Autodesk Inventor part; units mm, degrees
ref_plane "YZ Plane" through (0, 0, 0) normal (1, 0, 0) x (0, 1, 0)
ref_plane "XZ Plane" through (0, 0, 0) normal (0, 1, 0) x (-1, 0, 0)
ref_plane "XY Plane" through (0, 0, 0) normal (0, 0, 1) x (1, 0, 0)
sketch "Sketch1" plane through (0, 0, 0) normal (0, 0, 1) x (1, 0, 0)
  arc A0 (0, -0.381) -> (11, 10.619) centre (0, 10.619) ccw
  line L0 (11, 99.379) -> (11, 10.619)
  line L1 (0, -0.381) -> (-170.96, -0.381)
  arc A1 (11, 99.379) -> (0, 110.379) centre (0, 99.379) ccw
  line L2 (-170.96, 110.379) -> (0, 110.379)
  arc A2 (-170.96, 110.379) -> (-181.96, 99.379) centre (-170.96, 99.379) ccw
  line L3 (-181.96, 10.619) -> (-181.96, 99.379)
  arc A3 (-181.96, 10.619) -> (-170.96, -0.381) centre (-170.96, 10.619) ccw
  circle A4 centre (-22.38, 21.199) radius 1.5
  circle A5 centre (-148.58, 21.199) radius 1.5
  circle A6 centre (-148.58, 86.849) radius 1.5
  circle A7 centre (-22.38, 86.849) radius 1.5
  circle A8 centre (-22.38, 21.199) radius 1.905
  circle A9 centre (-22.38, 86.849) radius 1.905
  line L4 (-41.31, 1.719) -> (-129.65, 1.719)
  line L5 (-129.65, 108.279) -> (-41.31, 108.279)
  line L6 (8.9, 71.419) -> (8.9, 36.009)
  line L7 (-34.96, 23.309) -> (-34.96, 8.069)
  line L8 (-28.61, 29.659) -> (2.55, 29.659)
  arc A10 (-28.61, 29.659) -> (-34.96, 23.309) centre (-28.61, 23.309) ccw
  line L9 (2.55, 77.769) -> (-28.61, 77.769)
  line L10 (-34.96, 84.119) -> (-34.96, 101.929)
  arc A11 (-34.96, 84.119) -> (-28.61, 77.769) centre (-28.61, 84.119) ccw
  arc A12 (2.55, 29.659) -> (8.9, 36.009) centre (2.55, 36.009) ccw
  arc A13 (-41.31, 1.719) -> (-34.96, 8.069) centre (-41.31, 8.069) ccw
  arc A14 (-34.96, 101.929) -> (-41.31, 108.279) centre (-41.31, 101.929) ccw
  arc A15 (8.9, 71.419) -> (2.55, 77.769) centre (2.55, 71.419) ccw
  line L11 (-29.88, 25.199) -> (-29.88, 17.199)
  line L12 (-14.88, 25.199) -> (-29.88, 25.199)
  line L13 (-29.88, 82.849) -> (-14.88, 82.849)
  line L14 (-29.88, 90.849) -> (-29.88, 82.849)
  circle A16 centre (-148.58, 21.199) radius 1.905
  circle A17 centre (-148.58, 86.849) radius 1.905
  line L15 (-179.86, 71.419) -> (-179.86, 36.009)
  line L16 (-136, 23.309) -> (-136, 8.069)
  line L17 (-142.35, 29.659) -> (-173.51, 29.659)
  arc A18 (-136, 23.309) -> (-142.35, 29.659) centre (-142.35, 23.309) ccw
  line L18 (-173.51, 77.769) -> (-142.35, 77.769)
  line L19 (-136, 84.119) -> (-136, 101.929)
  arc A19 (-142.35, 77.769) -> (-136, 84.119) centre (-142.35, 84.119) ccw
  arc A20 (-179.86, 36.009) -> (-173.51, 29.659) centre (-173.51, 36.009) ccw
  arc A21 (-136, 8.069) -> (-129.65, 1.719) centre (-129.65, 8.069) ccw
  arc A22 (-129.65, 108.279) -> (-136, 101.929) centre (-129.65, 101.929) ccw
  arc A23 (-173.51, 77.769) -> (-179.86, 71.419) centre (-173.51, 71.419) ccw
  point P0 (0, 0)
  point P1 (-34.96, 1.719)
  point P2 (8.9, 29.659)
  point P3 (8.9, 77.769)
  point P4 (-34.96, 77.769)
  point P5 (-34.96, 108.279)
  dimension "d1" = 23.53
  dimension "d2" = 3.81
  dimension "d5" = 3.81
  dimension "d16" = 27.94
  dimension "d18" = 6.35
  dimension "d21" = 6.35
  dimension "d22" = 6.35
  dimension "d23" = 2.1
  dimension "d24" = 2.1
  dimension "d25" = 2.1
  dimension "d33" = 5.08
  dimension "d34" = 5.08
  dimension "d35" = 5.08
  dimension "d36" = 6.35
  dimension "d37" = 6.35
extrude "Extrusion3" add sketch "Sketch1" along normal blind 2.1 contours L1 A3 L3 A2 L2 A1 L0 A0
sketch "Sketch4" plane through (0, 0, 2.1) normal (0, 0, 1) x (1, 0, 0)
  arc A0 (-28.61, 29.659) -> (-34.96, 23.309) centre (-28.61, 23.309) ccw
  line L0 (-34.96, 23.309) -> (-34.96, 8.069)
  arc A1 (-41.31, 1.719) -> (-34.96, 8.069) centre (-41.31, 8.069) ccw
  line L1 (-41.31, 1.719) -> (-129.65, 1.719)
  arc A2 (-136, 8.069) -> (-129.65, 1.719) centre (-129.65, 8.069) ccw
  line L2 (-136, 8.069) -> (-136, 23.309)
  arc A3 (-136, 23.309) -> (-142.35, 29.659) centre (-142.35, 23.309) ccw
  line L3 (-142.35, 29.659) -> (-173.51, 29.659)
  arc A4 (-179.86, 36.009) -> (-173.51, 29.659) centre (-173.51, 36.009) ccw
  line L4 (-179.86, 36.009) -> (-179.86, 71.419)
  arc A5 (-173.51, 77.769) -> (-179.86, 71.419) centre (-173.51, 71.419) ccw
  line L5 (-173.51, 77.769) -> (-142.35, 77.769)
  arc A6 (-142.35, 77.769) -> (-136, 84.119) centre (-142.35, 84.119) ccw
  line L6 (-136, 84.119) -> (-136, 101.929)
  arc A7 (-129.65, 108.279) -> (-136, 101.929) centre (-129.65, 101.929) ccw
  line L7 (-129.65, 108.279) -> (-41.31, 108.279)
  arc A8 (-34.96, 101.929) -> (-41.31, 108.279) centre (-41.31, 101.929) ccw
  line L8 (-34.96, 101.929) -> (-34.96, 84.119)
  arc A9 (-34.96, 84.119) -> (-28.61, 77.769) centre (-28.61, 84.119) ccw
  line L9 (-28.61, 77.769) -> (2.55, 77.769)
  arc A10 (8.9, 71.419) -> (2.55, 77.769) centre (2.55, 71.419) ccw
  line L10 (8.9, 71.419) -> (8.9, 36.009)
  arc A11 (2.55, 29.659) -> (8.9, 36.009) centre (2.55, 36.009) ccw
  line L11 (2.55, 29.659) -> (-28.61, 29.659)
  circle A12 centre (-148.58, 86.849) radius 1.905
  circle A13 centre (-148.58, 21.199) radius 1.905
  circle A14 centre (-22.38, 86.849) radius 1.905
  circle A15 centre (-22.38, 21.199) radius 1.905
  arc A16 (0, -0.381) -> (11, 10.619) centre (0, 10.619) ccw
  line L12 (11, 10.619) -> (11, 99.379)
  arc A17 (11, 99.379) -> (0, 110.379) centre (0, 99.379) ccw
  line L13 (0, 110.379) -> (-170.96, 110.379)
  arc A18 (-170.96, 110.379) -> (-181.96, 99.379) centre (-170.96, 99.379) ccw
  line L14 (-181.96, 99.379) -> (-181.96, 10.619)
  arc A19 (-181.96, 10.619) -> (-170.96, -0.381) centre (-170.96, 10.619) ccw
  line L15 (-170.96, -0.381) -> (0, -0.381)
  arc A20 (0, 1.719) -> (8.9, 10.619) centre (0, 10.619) ccw
  line L16 (8.9, 10.619) -> (8.9, 99.379)
  arc A21 (8.9, 99.379) -> (0, 108.279) centre (0, 99.379) ccw
  line L17 (0, 108.279) -> (-170.96, 108.279)
  arc A22 (-170.96, 108.279) -> (-179.86, 99.379) centre (-170.96, 99.379) ccw
  line L18 (-179.86, 99.379) -> (-179.86, 10.619)
  arc A23 (-179.86, 10.619) -> (-170.96, 1.719) centre (-170.96, 10.619) ccw
  line L19 (-170.96, 1.719) -> (0, 1.719)
  point P0 (0, 0)
  dimension "d40" = 2.1
extrude "Extrusion4" add sketch "Sketch4" along normal blind 8.5 contours L15 A19 L14 A18 L13 A17 L12 A16
ref_plane "Work Plane1" through (-85.48, 10.619, 10.6) normal (-1, 0, 0) x (0, 0, 1)
ref_plane "Work Plane2" through (-170.96, 54.999, 10.6) normal (0, -1, 0) x (1, 0, 0)
sketch "Sketch9" plane through (0, 0, 0) normal (0, 0, -1) x (-1, 0, 0)
  arc A0 (-8.9, 10.619) -> (0, 1.719) centre (0, 10.619) ccw
  arc A1 (-6.8, 10.619) -> (0, 3.819) centre (0, 10.619) ccw
  line L0 (0, 1.719) -> (0, 3.819)
  line L1 (-6.8, 10.619) -> (-8.9, 10.619)
  arc A2 (170.96, 1.719) -> (179.86, 10.619) centre (170.96, 10.619) ccw
  arc A3 (170.96, 3.819) -> (177.76, 10.619) centre (170.96, 10.619) ccw
  line L2 (170.96, 3.819) -> (170.96, 1.719)
  line L3 (179.86, 10.619) -> (177.76, 10.619)
  arc A4 (179.86, 99.379) -> (170.96, 108.279) centre (170.96, 99.379) ccw
  arc A5 (177.76, 99.379) -> (170.96, 106.179) centre (170.96, 99.379) ccw
  line L4 (177.76, 99.379) -> (179.86, 99.379)
  line L5 (170.96, 108.279) -> (170.96, 106.179)
  arc A6 (0, 106.179) -> (-6.8, 99.379) centre (0, 99.379) ccw
  arc A7 (0, 108.279) -> (-8.9, 99.379) centre (0, 99.379) ccw
  line L6 (-8.9, 99.379) -> (-6.8, 99.379)
  line L7 (0, 106.179) -> (0, 108.279)
  line L8 (170.96, 1.719) -> (0, 1.719)
  line L9 (0.508, 1.719) -> (0, 1.719)
  line L10 (-6.36, 11.127) -> (-8.9, 11.127)
  line L11 (-8.9, 11.127) -> (-8.9, 10.619)
  line L12 (0.508, 1.719) -> (0.508, 4.259)
  arc A8 (-6.36, 11.127) -> (0.508, 4.259) centre (0.748, 11.367) ccw
  arc A9 (-8.9, 10.619) -> (0, 1.719) centre (0, 10.619) ccw
  line L13 (-6.36, 98.871) -> (-8.9, 98.871)
  line L14 (-8.9, 99.379) -> (-8.9, 10.619)
  line L15 (0.508, 105.739) -> (0.508, 108.279)
  line L16 (0.508, 108.279) -> (0, 108.279)
  arc A10 (0, 108.279) -> (-8.9, 98.871) centre (0, 99.3653) ccw
  arc A11 (0.508, 105.739) -> (-6.36, 98.871) centre (0.748, 98.631) ccw
  line L17 (0, -0.381) -> (170.96, -0.381)
  line L18 (85.48, -0.381) -> (85.48, 110.379)
  line L19 (170.96, 110.379) -> (0, 110.379)
  arc A12 (170.96, 1.719) -> (179.86, 10.619) centre (170.96, 10.619) ccw
  line L20 (170.452, 1.719) -> (170.96, 1.719)
  line L21 (177.32, 11.127) -> (179.86, 11.127)
  line L22 (170.452, 1.719) -> (170.452, 4.259)
  arc A13 (170.452, 4.259) -> (177.32, 11.127) centre (170.212, 11.367) ccw
  line L23 (177.32, 98.871) -> (179.86, 98.871)
  line L24 (179.86, 99.379) -> (179.86, 10.619)
  line L25 (170.452, 105.739) -> (170.452, 108.279)
  line L26 (170.452, 108.279) -> (170.96, 108.279)
  arc A14 (179.86, 98.871) -> (170.96, 108.279) centre (170.96, 99.3653) ccw
  arc A15 (177.32, 98.871) -> (170.452, 105.739) centre (170.212, 98.631) ccw
  point P0 (0, 0)
  point P1 (17.526, 1.719)
  dimension "d73" = 0.508
  dimension "d74" = 0.508
  dimension "d75" = 2.54
  dimension "d76" = 2.54
  dimension "d77" = 7.112
  dimension "d78" = 2.54
  dimension "d79" = 2.54
  dimension "d80" = 0.508
  dimension "d81" = 0.508
  dimension "d82" = 7.112
extrude "Extrusion7" cut sketch "Sketch9" against normal up to next contours L1 A1 L0 A0 | L7 A6 L6 A7 | A10 L16 L15 A11 L13 | L23 A15 L25 L26 L5 A5 L4 L24 | L24 A4 A14 | L22 A13 L21 L24 L3 A3 L2 L8 | L2 A3 L3 A2 | L4 A5 L5 A4
sketch "Sketch10" plane through (0, 0, 0) normal (0, 0, -1) x (-1, 0, 0)
  line L0 (-3.38, 18.0763) -> (14.4, 27.559)
  line L1 (14.4, 27.559) -> (-3.38, 27.559)
  line L2 (-3.38, 27.559) -> (-3.38, 18.0763)
  line L3 (10.7529, 7.239) -> (29.8029, 17.399)
  line L4 (29.8029, 17.399) -> (29.8029, 7.239)
  line L5 (29.8029, 7.239) -> (10.7529, 7.239)
  line L6 (0, -0.381) -> (170.96, -0.381)
  line L7 (-11, 99.379) -> (-11, 10.619)
  line L8 (181.96, 99.379) -> (181.96, 10.619)
  line L9 (181.96, 54.999) -> (-11, 54.999)
  line L10 (-11, 10.619) -> (-11, 99.379)
  line L11 (85.48, -0.381) -> (85.48, 110.379)
  line L12 (0, 110.379) -> (170.96, 110.379)
  line L13 (174.34, 18.0763) -> (156.56, 27.559)
  line L14 (156.56, 27.559) -> (174.34, 27.559)
  line L15 (174.34, 27.559) -> (174.34, 18.0763)
  line L16 (160.2071, 7.239) -> (141.1571, 17.399)
  line L17 (141.1571, 17.399) -> (141.1571, 7.239)
  line L18 (141.1571, 7.239) -> (160.2071, 7.239)
  line L19 (-3.38, 91.9217) -> (14.4, 82.439)
  line L20 (14.4, 82.439) -> (-3.38, 82.439)
  line L21 (-3.38, 82.439) -> (-3.38, 91.9217)
  line L22 (10.7529, 102.759) -> (29.8029, 92.599)
  line L23 (29.8029, 92.599) -> (29.8029, 102.759)
  line L24 (29.8029, 102.759) -> (10.7529, 102.759)
  line L25 (141.1571, 102.759) -> (160.2071, 102.759)
  line L26 (141.1571, 92.599) -> (141.1571, 102.759)
  line L27 (160.2071, 102.759) -> (141.1571, 92.599)
  line L28 (174.34, 91.9217) -> (156.56, 82.439)
  line L29 (156.56, 82.439) -> (174.34, 82.439)
  line L30 (174.34, 82.439) -> (174.34, 91.9217)
  point P0 (0, 0)
  point P1 (-11, 19.255)
  dimension "d85" = 17.78
  dimension "d86" = 19.05
  dimension "d87" = 10.16
  dimension "d88" = 7.62
  dimension "d89" = 7.62
  dimension "d102" = 27.94
extrude "Extrusion8" cut sketch "Sketch10" against normal up to next
sketch "Sketch11" plane through (0, 0, 2.1) normal (0, 0, 1) x (1, 0, 0)
  arc A0 (-144.389, 84.944) -> (-144.389, 88.754) centre (-144.389, 86.849) ccw
  circle A1 centre (-148.58, 86.849) radius 1.905
  arc A2 (-152.771, 88.754) -> (-152.771, 84.944) centre (-152.771, 86.849) ccw
  line L0 (-152.771, 88.754) -> (-144.389, 88.754)
  line L1 (-144.389, 84.944) -> (-152.771, 84.944)
  circle A3 centre (-148.58, 21.199) radius 1.905
  arc A4 (-144.389, 19.294) -> (-144.389, 23.104) centre (-144.389, 21.199) ccw
  arc A5 (-152.771, 23.104) -> (-152.771, 19.294) centre (-152.771, 21.199) ccw
  line L2 (-152.771, 23.104) -> (-144.389, 23.104)
  line L3 (-152.771, 19.294) -> (-144.389, 19.294)
  line L4 (-85.48, -22.533) -> (-85.48, 132.531)
  arc A6 (-26.571, 88.754) -> (-26.571, 84.944) centre (-26.571, 86.849) ccw
  arc A7 (-18.189, 84.944) -> (-18.189, 88.754) centre (-18.189, 86.849) ccw
  line L5 (-18.189, 88.754) -> (-26.571, 88.754)
  line L6 (-26.571, 84.944) -> (-18.189, 84.944)
  arc A8 (-26.571, 23.104) -> (-26.571, 19.294) centre (-26.571, 21.199) ccw
  arc A9 (-18.189, 19.294) -> (-18.189, 23.104) centre (-18.189, 21.199) ccw
  line L7 (-18.189, 23.104) -> (-26.571, 23.104)
  line L8 (-18.189, 19.294) -> (-26.571, 19.294)
  point P0 (0, 0)
  point P1 (-148.58, 88.754)
  point P2 (-148.58, 23.104)
  dimension "d92" = 3.81
  dimension "d93" = 1.905
  dimension "d94" = 1.905
  dimension "d96" = 8.382
  dimension "d97" = 1.905
  dimension "d98" = 1.905
  dimension "d101" = 8.382
extrude "Extrusion9" cut sketch "Sketch11" against normal up to next contours L1 A1 L0 A0 | L1 A2 L0 A1 | A3 L2 A4 L3 | A3 L3 A5 L2 | L5 A7 L6 A6 | L7 A9 L8 A8
equation "\"d24\" = d23"
equation "\"d25\" = d23"
equation "\"d36\" = d22"
equation "\"d37\" = d22"
equation "\"d74\" = d73"
equation "\"d76\" = d75"
equation "\"d78\" = d75"
equation "\"d79\" = d78"
equation "\"d80\" = d74"
equation "\"d81\" = d80"
equation "\"d82\" = d77"
equation "\"d93\" = 0.5 * d92"
equation "\"d94\" = 0.5 * d95"
equation "\"d97\" = d93"
equation "\"d98\" = d99"
equation "\"d101\" = d96"
equation "\"d99\" = 0.5 * d100"
properties part number "Hub Enclosure Front (new)"
The listing builds one solid part. Answer for the finished solid, in the listing's coordinates (mm). A direction names the side the tool comes from. Round coordinates to 2 decimals unless told otherwise and drop trailing zeros. Write each loop counter-clockwise with the first axis right and the second up, starting at its lowest first coordinate (ties: lowest second). Pieces come first, ordered by that corner, then holes. Notation, with made-up numbers: M 80.5,34.5 L 100.5,34.5 A20 cw 100.5,39.5 Z; hole C 54.25,78 d11. An arc over 180 degrees is marked long. Write each question's results on one line, items separated by ' | '. Start each with the question number.
Item 1: Flat-ended cylindrical pins translate along their axes: pin 1 Ø0.6 at (y, z) = (2.5, 1.5) entering from +X; pin 2 Ø8 at (x, y) = (-144.5, 30.5) entering from +Z; pin 3 Ø1 at (x, z) = (-178, 1.5) entering from -Y. Find the tip coordinate at first contact, or state that the pin passes through.
Item 2: A cutting plane is placed at D-D on x = -7.5. Write down the section's boundary in (y, z), and give its area (3 significant figures).
Item 3: For faces 4 (the face through (7.863, 2.927, 5.226)), 5 (the face through (-11, 90, 2.1)), 6 (the face through (-134.09, 3.53, 1.04)), determine the directions among +Z, -Z, +X, -X, +Y, -Y from which every point of the face is accessible in a straight line to the end or side of a thin tool.
Item 4: A cutting plane is placed at C-C on z = 8.5. Write down the section's boundary in (x, y), and give its area (3 significant figures).
Item 5: For a pull along Y with two mould halves and no side action, classify faces 1 (the face through (-84, -0.381, 5)), 2 (the face through (-36.8, 3.6, 1)), 3 (the face through (11, 56, 5)) as pulls with the +Y half, pulls with the -Y half, needs draft (parallel to the pull), parting line crosses it, or undercut.
Item 6: A cutting plane is placed at B-B on x = -69. Write down the section's boundary in (y, z), and give its area (3 significant figures).
Item 7: Straight lines are drawn through the part: L1, parallel to X at y = 89.5, z = 9.75; L2, parallel to Y at x = -89, z = 4.5; L3, parallel to X at y = 85.5, z = 1.75. For each, find the intervals that lie inside material, in ascending order. Write a range as [from, to].
Item 8: A cutting plane is placed at A-A on y = 52. Write down the section's boundary in (x, z), and give its area (3 significant figures).
Check sheet entries:
1) pin 1: x = 7.74 | pin 2: z = 2.1 | pin 3: y = 1.77
2) outline: M -0.38,0 L 23.88,0 L 23.88,2.1 L 1.72,2.1 L 1.72,10.6 L -0.38,10.6 Z; M 27.56,0 L 29.66,0 L 29.66,2.1 L 27.56,2.1 Z; M 77.77,0 L 82.44,0 L 82.44,2.1 L 77.77,2.1 Z; M 86.12,0 L 110.38,0 L 110.38,10.6 L 108.28,10.6 L 108.28,2.1 L 86.12,2.1 Z | area: 152 mm²
3) face 4: +Z, -Z, +X, -Y | face 5: +Z | face 6: +Z, -Z
4) outline: M -181.96,10.62 A11 ccw -170.96,-0.38 L 0,-0.38 A11 ccw 11,10.62 L 11,99.38 A11 ccw 0,110.38 L -170.96,110.38 A11 ccw -181.96,99.38 Z; hole M -179.86,10.62 A8.9 ccw -170.96,1.72 L 0,1.72 A8.9 ccw 8.9,10.62 L 8.9,98.87 A8.91 ccw 0,108.28 L -170.96,108.28 A8.91 ccw -179.86,98.87 Z | area: 1,220 mm²
5) face 1: pulls with the -Y half | face 2: undercut | face 3: needs draft
6) outline: M -0.38,0 L 1.72,0 L 1.72,10.6 L -0.38,10.6 Z; M 108.28,0 L 110.38,0 L 110.38,10.6 L 108.28,10.6 Z | area: 44.5 mm²
7) L1: [-181.96, -179.86], [8.9, 11] | L2: [-0.38, 1.72], [108.28, 110.38] | L3: [-181.96, -174.34], [-162.3, -154.12], [-143.04, -136], [-34.96, -27.92], [-16.84, -8.66], [3.38, 11]
8) outline: M -181.96,0 L -179.86,0 L -179.86,10.6 L -181.96,10.6 Z; M 8.9,0 L 11,0 L 11,10.6 L 8.9,10.6 Z | area: 44.5 mm²
